from build123d import *

# Parameters (mm, degrees)
F0_R     = 42.000965
F1_DEPTH = 19.05
F2_DEPTH = 0.029528
F3_T     = -2.54


with BuildPart() as f1:
    # F0 (on Top) → F1 (new body)
    with BuildSketch(Plane.XY):
        Circle(F0_R)
    extrude(amount=F1_DEPTH)

    # F3
    f3_openings = [f1.faces().sort_by_distance(p)[0] for p in [
        (0, 0, 19.05),
    ]]
    offset(amount=F3_T, openings=f3_openings)


with BuildPart() as f2:
    # F0 (on Top) → F2 (new body)
    with BuildSketch(Plane.XY):
        Circle(F0_R)
    extrude(amount=F2_DEPTH)


solid = f1.part
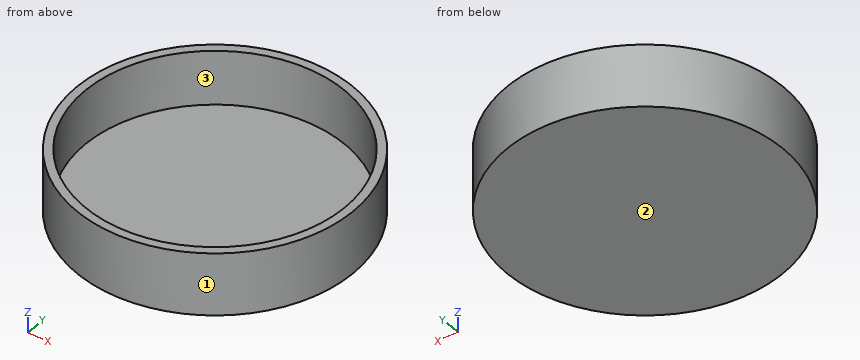
Input: part model. Units: mm. Frame: model coordinates. Face numbers are marked on the shaded views. Give positions to 0.01 mm unless a question says otherwise; leave off trailing zeros. Write each loop counter-clockwise with the first axis right and the second up, starting at its lowest first coordinate (ties: lowest second). Pieces come first, ordered by that corner, then holes. Notation, with made-up numbers: M -39,40 L -11,40 A16 ccw -11,58 Z; hole C 14,82 d9. An arc over 180 degrees is marked long. Use one line per item in the form item = value.
1. Cut plane A-A on y = 0. Return loops of the section in (x, z), and give its area (3 significant figures).
Outcome:
outline = M -42,0 L 42,0 L 42,19.05 L 39.46,19.05 L 39.46,2.54 L -39.46,2.54 L -39.46,19.05 L -42,19.05 Z
area = 297 mm²
2. First-contact query: P1, Ø6, axis at x = -5, y = 22.5, coming from the +Z side; P2, Ø6, axis at x = -5.5, y = 24, coming from the -Z side; P3, Ø1.5, axis at y = -3, z = 11.5, coming from the -X side; P4, Ø8, axis at x = -3.5, z = 3.5, coming from the -Y side. Flat tips, straight axial feed; report the tip coordinate or a pass-through.
Outcome:
P1 = 2.54
P2 = 0
P3 = -41.94
P4 = -42
3. Cut plane C-C on z = 17.5. Return loops of the section in (x, y), and give its area (3 significant figures).
Outcome:
outline = C 0,0 d84; hole C 0,0 d78.92
area = 650 mm²
4. Ray query, L1, parallel to Y at x = 0, z = 10.5; L2, parallel to Z at x = 19, y = -10.5; L3, parallel to X at y = 30, z = 4. Return the intervals inside material, ascending.
Outcome:
L1 = -42 to -39.46, 39.46 to 42
L2 = 0 to 2.54
L3 = -29.4 to -25.64, 25.64 to 29.4
5. Mould query, pull axis X, two halves, no side actions, for the marked faces 1, 2 and 3. Classes: released by +X, released by -X, zero draft, split by the parting line, or undercut.
Outcome:
face_1 = split by the parting line
face_2 = zero draft
face_3 = undercut
6. Cut plane D-D on z = 1. Return loops of the section in (x, y), and give its area (3 significant figures).
Outcome:
outline = C 0,0 d84
area = 5,540 mm²
